CAD build for the part. Positions are in the model's coordinates, mm. Face numbers are marked on the shaded views. Coordinates: 2 decimals unless noted, no trailing zeros. Write each loop counter-clockwise with the first axis right and the second up, starting at its lowest first coordinate (ties: lowest second). Pieces come first, ordered by that corner, then holes. Notation, with made-up numbers: (88.5, 54) -> (128.5, 54) arc R12 cw to (128.5, 62) -> close; hole circle Ø1 at (-26.5, 6). An arc over 180 degrees is marked (long way). Answer as CSV lines item,"result".
```python
from build123d import *

# Parameters (mm, degrees)
F1_DEPTH = 12
F2_T     = -3
F4_DEPTH = 3
F5_R     = 1
F6_W     = 32
F6_H     = 19
F6_W_2   = 30
F6_H_2   = 17
F7_DEPTH = 1
F9_DEPTH = 1
F10_R    = 1


with BuildPart() as f1:
    # F0 (on Top) → F1 (new body)
    with BuildSketch(Plane.XY):
        with BuildLine():
            Line((-24, -16.25), (19, -16.25))
            ThreePointArc((19, -16.25), (22.7217369359, -8.5009191815), (24, -2.376e-07))
            ThreePointArc((24, -2.376e-07), (22.7217370058, 8.5009189544), (19, 16.25))
            Line((19, 16.25), (-24, 16.25))
            Line((-24, 16.25), (-24, -16.25))
        make_face()
    extrude(amount=F1_DEPTH)

    # F2
    f2_openings = [f1.faces().sort_by_distance(p)[0] for p in [
        (-24, 0, 6),
    ]]
    offset(amount=F2_T, openings=f2_openings)

    # F3 (on face) → F4 (cut, through all)
    with BuildSketch(Plane.XY.offset(12)):
        with BuildLine():
            ThreePointArc((-8, 12.5), (-11.9542437084, 11.0126440912), (-13.9480315021, 7.2879855647))
            Line((-13.9480315021, 7.2879855647), (-2, 6.4416666667))
            Line((-2, 6.4416666667), (-2, 6.5))
            ThreePointArc((-2, 6.5), (-3.7573593129, 10.7426406871), (-8, 12.5))
        make_face()
        with BuildLine():
            Line((-2, 6.4416666667), (-13.9480315021, 7.2879855647))
            ThreePointArc((-13.9480315021, 7.2879855647), (-13.9869937787, 6.8948486973), (-14, 6.5))
            Line((-14, 6.5), (-14, -6.5))
            ThreePointArc((-14, -6.5), (-13.9869937787, -6.8948486973), (-13.9480315021, -7.2879855647))
            Line((-13.9480315021, -7.2879855647), (-2, -6.4416666667))
            Line((-2, -6.4416666667), (-2, 6.4416666667))
        make_face()
        with BuildLine():
            Line((-2, -6.4416666667), (-13.9480315021, -7.2879855647))
            ThreePointArc((-13.9480315021, -7.2879855647), (-11.9542437084, -11.0126440912), (-8, -12.5))
            ThreePointArc((-8, -12.5), (-3.7573593129, -10.7426406871), (-2, -6.5))
            Line((-2, -6.5), (-2, -6.4416666667))
        make_face()
        with BuildLine():
            Line((-13.9480315021, 7.2879855647), (-24, 8))
            Line((-24, 8), (-24, -8))
            Line((-24, -8), (-13.9480315021, -7.2879855647))
            ThreePointArc((-13.9480315021, -7.2879855647), (-13.9869937787, -6.8948486973), (-14, -6.5))
            Line((-14, -6.5), (-14, 6.5))
            ThreePointArc((-14, 6.5), (-13.9869937787, 6.8948486973), (-13.9480315021, 7.2879855647))
        make_face()
        Polygon((0, 6.3), (-2, 6.4416666667), (-2, -6.4416666667), (0, -6.3), (0, 0), align=None)
    extrude(amount=-F4_DEPTH, mode=Mode.SUBTRACT)

    # F5
    f5_edges = [f1.edges().sort_by_distance(p)[0] for p in [
        (0, 6.3, 10.5),
        (0, -6.3, 10.5),
    ]]
    fillet(f5_edges, radius=F5_R)

    # F6 (on face) → F7 (cut)
    with BuildSketch(Plane(origin=(0, 0, 0), x_dir=(1, 0, 0), z_dir=(0, 0, -1))):
        Rectangle(F6_W, F6_H)
        Rectangle(F6_W_2, F6_H_2, mode=Mode.SUBTRACT)
    extrude(amount=-F7_DEPTH, mode=Mode.SUBTRACT)

    # F8 (on face) → F9 (join)
    with BuildSketch(Plane(origin=(0, 0, 9), x_dir=(1, 0, 0), z_dir=(0, 0, -1))):
        with BuildLine():
            ThreePointArc((-4.3342804253, 11.25), (-8, 12.5), (-11.6657195747, 11.25))
            Line((-11.6657195747, 11.25), (-4.3342804253, 11.25))
        make_face()
        with BuildLine():
            Line((-4.3342804253, -11.25), (-11.6657195747, -11.25))
            ThreePointArc((-11.6657195747, -11.25), (-8, -12.5), (-4.3342804253, -11.25))
        make_face()
        with BuildLine():
            Line((-24, -11.25), (-24, -13.25))
            Line((-24, -13.25), (17.355180526, -13.25))
            ThreePointArc((17.355180526, -13.25), (21, 0), (17.355180526, 13.25))
            Line((17.355180526, 13.25), (-24, 13.25))
            Line((-24, 13.25), (-24, 11.25))
            Line((-24, 11.25), (-11.6657195747, 11.25))
            ThreePointArc((-11.6657195747, 11.25), (-8, 12.5), (-4.3342804253, 11.25))
            Line((-4.3342804253, 11.25), (2, 11.25))
            Line((2, 11.25), (2, -11.25))
            Line((2, -11.25), (-4.3342804253, -11.25))
            ThreePointArc((-4.3342804253, -11.25), (-8, -12.5), (-11.6657195747, -11.25))
            Line((-11.6657195747, -11.25), (-24, -11.25))
        make_face()
    extrude(amount=F9_DEPTH)

    # F10
    f10_edges = [f1.edges().sort_by_distance(p)[0] for p in [
        (-2.5, -16.25, 12),
        (24, 0, 12),
        (-2.5, 16.25, 12),
        (19, -16.25, 6),
        (19, 16.25, 6),
        (24, 0, 0),
        (-2.5, 16.25, 0),
        (-2.5, -16.25, 0),
        (-24, -16.25, 6),
        (-24, -12.125, 12),
        (-24, 0, 0),
        (-24, 12.125, 12),
        (-24, 16.25, 6),
    ]]
    fillet(f10_edges, radius=F10_R)


solid = f1.part
```
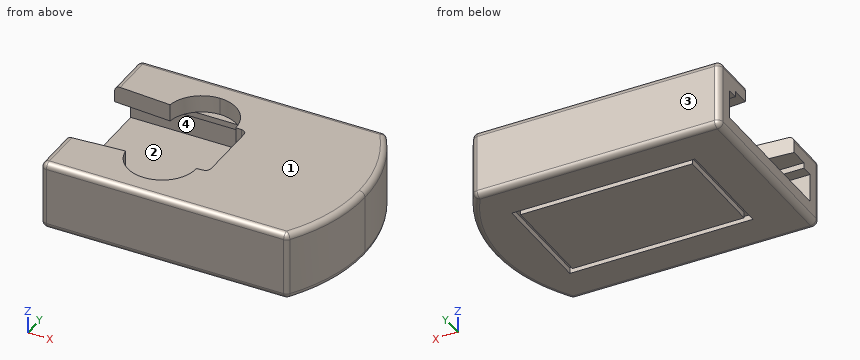
Item 1: Saw through at C-C on x = -6.5. Give the cut face in (y, z), and give its area (3 significant figures).
Answer below:
outline,"(-16.25, 1) arc R1 ccw to (-15.25, 0) -> (-9.5, 0) -> (-9.5, 1) -> (-8.5, 1) -> (-8.5, 0) -> (8.5, 0) -> (8.5, 1) -> (9.5, 1) -> (9.5, 0) -> (15.25, 0) arc R1 ccw to (16.25, 1) -> (16.25, 11) arc R1 ccw to (15.25, 12) -> (12.31, 12) -> (12.31, 9) -> (11.25, 9) -> (11.25, 8) -> (13.25, 8) -> (13.25, 3) -> (-13.25, 3) -> (-13.25, 8) -> (-11.25, 8) -> (-11.25, 9) -> (-12.31, 9) -> (-12.31, 12) -> (-15.25, 12) arc R1 ccw to (-16.25, 11) -> close"
area,"158 mm2"
Item 2: Flat gauge pins, fed straight in: pin 1 (0.5 mm diameter, centred on y = -4, z = 0.5, fed in from -X); pin 2 (1.5 mm diameter, centred on y = -1, z = 10.5, fed in from -X); pin 3 (1 mm diameter, centred on x = -8, y = -11.5, fed in from +Z). Where does each tip first touch, or does it go through?
Answer below:
pin 1,"stops at x = -23.97"
pin 2,"stops at x = 0"
pin 3,"stops at z = 9"
Item 3: Saw through at A-A on x = 10.5. Give the cut face in (y, z).
Answer below:
outline,"(-16.25, 1) arc R1 ccw to (-15.25, 0) -> (-9.5, 0) -> (-9.5, 1) -> (-8.5, 1) -> (-8.5, 0) -> (8.5, 0) -> (8.5, 1) -> (9.5, 1) -> (9.5, 0) -> (15.25, 0) arc R1 ccw to (16.25, 1) -> (16.25, 11) arc R1 ccw to (15.25, 12) -> (-15.25, 12) arc R1 ccw to (-16.25, 11) -> close; hole (-13.25, 3) -> (13.25, 3) -> (13.25, 8) -> (-13.25, 8) -> close"
Item 4: Two-plate mould, pull along Z, no slides. Class the marked faces 1, 2, 3 and 4: pulls with the +Z half, pulls with the -Z half, needs draft (parallel to the pull), parting line crosses it, or undercut.
Answer below:
face 1,"pulls with the +Z half"
face 2,"undercut"
face 3,"needs draft"
face 4,"undercut"
Item 5: Saw through at B-B on z = 5.75. Give the cut face in (x, y), and give its area (3 significant figures).
Answer below:
outline,"(-24, -15.25) arc R1 ccw to (-23, -16.25) -> (18.46, -16.25) arc R1 ccw to (19.3, -15.8) arc R28.91 ccw to (19.3, 15.8) arc R1 ccw to (18.46, 16.25) -> (-23, 16.25) arc R1 ccw to (-24, 15.25) -> (-24, 13.25) -> (17.36, 13.25) arc R25.91 cw to (17.36, -13.25) -> (-24, -13.25) -> close"
area,"346 mm2"
Item 6: Saw through at D-D on z = 10.5. Give the cut face in (x, y), and give its area (3 significant figures).
Answer below:
outline,"(-24, -15.25) arc R1 ccw to (-23, -16.25) -> (18.46, -16.25) arc R1 ccw to (19.3, -15.8) arc R28.91 ccw to (19.3, 15.8) arc R1 ccw to (18.46, 16.25) -> (-23, 16.25) arc R1 ccw to (-24, 15.25) -> (-24, 8) -> (-13.95, 7.29) arc R6 cw to (-2, 6.5) -> (-2, 6.44) -> (-0.93, 6.37) arc R1 cw to (0, 5.37) -> (0, -5.37) arc R1 cw to (-0.93, -6.37) -> (-2, -6.44) -> (-2, -6.5) arc R6 cw to (-13.95, -7.29) -> (-24, -8) -> close"
area,"1,060 mm2"
Item 7: Wall check: line 1 (Y direction, x = -1, z = 7); line 2 (X direction, y = 5.5, z = 0.5). Give the ranges that are in metal, low to high. Write a range as from..to.
Answer below:
line 1,"y = -16.25..-13.25, 13.25..16.25"
line 2,"x = -23.87..-16, -15..15, 16..23.34"
